```python
from build123d import *

# Parameters (mm, degrees)
F0_W          = 69.85
F0_H          = 69.85
F1_DEPTH      = 3.175
F2_R          = 3.175
F3_R          = 1.7499965
F4_DEPTH      = 25.4
F4_DEPTH_BACK = 101
F6_DEPTH      = 25.4
F7_R          = 1.499997
F8_DEPTH      = 6.35
F10_W         = 44.45
F10_H         = 57.15
F11_DEPTH     = 1.27
F12_W         = 8.9916
F12_H         = 14.4018
F13_DEPTH     = 10.9982


# Not quite as in the source:
# - an extrude ends at something that could not be found from the text; its depth is read off the source's solid


with BuildPart() as f1:
    # F0 (on Top) → F1 (new body)
    with BuildSketch(Plane.XY):
        Rectangle(F0_W, F0_H)
    extrude(amount=F1_DEPTH)

    # F2
    f2_edges = [f1.edges().sort_by_distance(p)[0] for p in [
        (-34.925, -34.925, 1.5875),
        (34.925, -34.925, 1.5875),
        (34.925, 34.925, 1.5875),
        (-34.925, 34.925, 1.5875),
    ]]
    fillet(f2_edges, radius=F2_R)

    # F3 (on face) → F4 (cut, two sides)
    with BuildSketch(Plane.XY.offset(3.175)) as f4_sk:
        with Locations((-31.75, 31.75)):
            Circle(F3_R)
        with Locations((31.75, 31.75)):
            Circle(F3_R)
        with Locations((31.75, -31.75)):
            Circle(F3_R)
        with Locations((-31.75, -31.75)):
            Circle(F3_R)
    extrude(amount=-F4_DEPTH, mode=Mode.SUBTRACT)
    extrude(f4_sk.sketch, amount=F4_DEPTH_BACK, mode=Mode.SUBTRACT)

    # F5 (on face) → F6 (join)
    with BuildSketch(Plane.XY.offset(3.175)):
        with BuildLine():
            Line((25.4, 34.925), (-25.4, 34.925))
            ThreePointArc((-25.4, 34.925), (-27.6450640303, 33.9950640303), (-28.575, 31.75))
            Line((-28.575, 31.75), (-28.575, -31.75))
            ThreePointArc((-28.575, -31.75), (-27.6450640303, -33.9950640303), (-25.4, -34.925))
            Line((-25.4, -34.925), (25.4, -34.925))
            ThreePointArc((25.4, -34.925), (27.6450640303, -33.9950640303), (28.575, -31.75))
            Line((28.575, -31.75), (28.575, 31.75))
            ThreePointArc((28.575, 31.75), (27.6450640303, 33.9950640303), (25.4, 34.925))
        make_face()
        with BuildLine():
            ThreePointArc((-25.4, 28.575), (-23.1549359697, 29.5049359697), (-22.225, 31.75))
            Line((-22.225, 31.75), (22.225, 31.75))
            ThreePointArc((22.225, 31.75), (23.1549359697, 29.5049359697), (25.4, 28.575))
            Line((25.4, 28.575), (25.4, -28.575))
            ThreePointArc((25.4, -28.575), (23.1549359697, -29.5049359697), (22.225, -31.75))
            Line((22.225, -31.75), (-22.225, -31.75))
            ThreePointArc((-22.225, -31.75), (-23.1549359697, -29.5049359697), (-25.4, -28.575))
            Line((-25.4, -28.575), (-25.4, 28.575))
        make_face(mode=Mode.SUBTRACT)
    extrude(amount=F6_DEPTH)

    # F7 (on face) → F8 (cut)
    with BuildSketch(Plane.XY.offset(28.575)):
        with Locations((-25.4, 31.75)):
            Circle(F7_R)
        with Locations((25.4, 31.75)):
            Circle(F7_R)
        with Locations((25.4, -31.75)):
            Circle(F7_R)
        with Locations((-25.4, -31.75)):
            Circle(F7_R)
    extrude(amount=-F8_DEPTH, mode=Mode.SUBTRACT)


with BuildPart() as f11:
    # F10 (on offset) → F11 (new body)
    with BuildSketch(Plane.XY.offset(6.35)):
        with Locations((0.3046067432, 0.0383506862)):
            Rectangle(F10_W, F10_H)
    extrude(amount=F11_DEPTH)

    # F12 (on face) → F13 (join)
    with BuildSketch(Plane.XY.offset(7.62)):
        with Locations((-12.7947921936, -21.3357493138)):
            Rectangle(F12_W, F12_H)
    extrude(amount=F13_DEPTH)


solid = f1.part
```
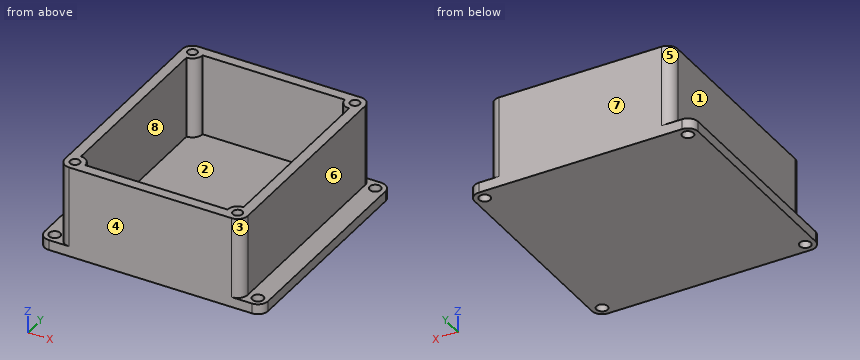
Source: CAD feature listing. Evaluate the final solid. Frame: model axes, mm. Face numbers are marked on the shaded views. A direction names the side the tool comes from. Coordinates: 2 decimals unless noted, no trailing zeros. Loops run counter-clockwise (first coordinate to the right, second up) from the corner with the lowest first, then second, coordinate; pieces in that order, holes last. Notation, with made-up numbers: M -33,12 L 16,12 A12 ccw 16,19 Z; hole C 35.25,-17.5 d3. An arc over 180 degrees is marked long. Put each result on its own line as item: value. Start each with the question number.
1) Ray query, L1, parallel to Y at x = 31.75, z = 2.25 (3 decimals); L2, parallel to X at y = 23, z = 24 (3 decimals); L3, parallel to Y at x = 21, z = 13.75 (3 decimals). Return the intervals inside material, ascending. Write a range as from..to.
2) Cut plane D-D on z = 21. Return the cut outline in (x, y) (3 decimals).
3) Pull-direction query (Y, two-part tool) for the marked faces 1, 2 and 3; classes: pulls with the +Y half, pulls with the -Y half, needs draft (parallel to the pull), parting line crosses it, or undercut.
4) Reachability of the marked faces 4, 5, 6, 7 and 8 from +Z, -Z, +X, -X, +Y, -Y: full face, straight path, thin tool, end or side. Return the list, or none.
5) Cut plane B-B on y = 24. Return the cut outline in (x, z) (3 decimals), then the cut area to 3 significant figures.
6) Cut plane A-A on z = 26.75. Return the cut outline in (x, y) (3 decimals).
7) Contact query for flat-ended pins moving along their axis: pin 1 Ø4 at (x, y) = (31.75, 31.75) entering from +Z (3 decimals); pin 2 Ø1.8 at (x, y) = (-25.4, 31.75) entering from +Z (3 decimals); pin 3 Ø5 at (x, y) = (30.5, 17) entering from +Z (3 decimals); pin 4 Ø3 at (x, y) = (-31.75, -31.75) entering from +Z. Output: stop coordinate, or through.
8) Cut plane C-C on x = 8. Return the cut outline in (y, z) (3 decimals), then the cut area to 3 significant figures.
The answers:
1. L1: y = -34.925..-33.5, -30..30, 33.5..34.925
1. L2: x = -28.575..-25.4, 25.4..28.575
1. L3: y = -34.925..-31.75, 31.75..34.925
2. outline: M -28.575,-31.75 A3.175 ccw -25.4,-34.925 L 25.4,-34.925 A3.175 ccw 28.575,-31.75 L 28.575,31.75 A3.175 ccw 25.4,34.925 L -25.4,34.925 A3.175 ccw -28.575,31.75 Z; hole M -25.4,-28.575 A3.175 cw -22.225,-31.75 L 22.225,-31.75 A3.175 cw 25.4,-28.575 L 25.4,28.575 A3.175 cw 22.225,31.75 L -22.225,31.75 A3.175 cw -25.4,28.575 Z
3. face 1: needs draft
3. face 2: undercut
3. face 3: pulls with the -Y half
4. face 4: +Z, -Z, +X, -X, -Y
4. face 5: +Z, -X, +Y
4. face 6: +Z, +X, +Y, -Y
4. face 7: +Z, -Z, +X, -X, +Y
4. face 8: +Z
5. outline: M -34.925,0 L 34.925,0 L 34.925,3.175 L 28.575,3.175 L 28.575,28.575 L 25.4,28.575 L 25.4,3.175 L -25.4,3.175 L -25.4,28.575 L -28.575,28.575 L -28.575,3.175 L -34.925,3.175 Z
5. area: 383 mm²
6. outline: M -28.575,-31.75 A3.175 ccw -25.4,-34.925 L 25.4,-34.925 A3.175 ccw 28.575,-31.75 L 28.575,31.75 A3.175 ccw 25.4,34.925 L -25.4,34.925 A3.175 ccw -28.575,31.75 Z; hole C -25.4,-31.75 d3; hole C -25.4,31.75 d3; hole M -25.4,-28.575 A3.175 cw -22.225,-31.75 L 22.225,-31.75 A3.175 cw 25.4,-28.575 L 25.4,28.575 A3.175 cw 22.225,31.75 L -22.225,31.75 A3.175 cw -25.4,28.575 Z; hole C 25.4,-31.75 d3; hole C 25.4,31.75 d3
7. pin 1: stops at z = 3.175
7. pin 2: stops at z = 22.225
7. pin 3: stops at z = 28.575
7. pin 4: passes through
8. outline: M -34.925,0 L 34.925,0 L 34.925,28.575 L 31.75,28.575 L 31.75,3.175 L -31.75,3.175 L -31.75,28.575 L -34.925,28.575 Z
8. area: 383 mm²
